from build123d import *

# Parameters (mm, degrees)
F0_R     = 35
F1_DEPTH = 25
F3_DEPTH = 5


with BuildPart() as f1:
    # F0 (on Top) → F1 (new body)
    with BuildSketch(Plane.XY):
        Circle(F0_R)
    extrude(amount=F1_DEPTH)

    # F2 (on face) → F3 (join)
    with BuildSketch(Plane(origin=(0, 0, 0), x_dir=(1, 0, 0), z_dir=(0, 0, -1))):
        with BuildLine():
            Line((-5, 22.5), (-5, 17.811513))
            ThreePointArc((-5, 17.811513), (-18.5, 0), (-5, -17.811513))
            Line((-5, -17.811513), (-5, -22.5))
            Line((-5, -22.5), (5, -22.5))
            Line((5, -22.5), (5, -17.811513))
            ThreePointArc((5, -17.811513), (18.5, 0), (5, 17.811513))
            Line((5, 17.811513), (5, 22.5))
            Line((5, 22.5), (-5, 22.5))
        make_face()
    extrude(amount=F3_DEPTH)


solid = f1.part
Part model, mm, in its own coordinate system. A direction names the side the tool comes from. Round coordinates to 2 decimals unless told otherwise and drop trailing zeros. Order: outer loops, then holes, each group sorted by start corner. A loop starts at its lowest first (then second) coordinate and runs counter-clockwise, first axis right, second up. Notation, with made-up numbers: (-33.5, -26.75) -> (-9.5, -26.75) arc R16 ccw to (-9.5, -20.75) -> close; hole circle Ø1 at (-27, 68). An arc over 180 degrees is marked (long way). Put each result on its own line as item: value.
Q1. Band-saw the part on A-A (x = 0). Give the cut face in (y, z).
From the geometry:
outline: (-35, 0) -> (-22.5, 0) -> (-22.5, -5) -> (22.5, -5) -> (22.5, 0) -> (35, 0) -> (35, 25) -> (-35, 25) -> close
Q2. Tool access for faces 1 (the face through (18.497, 0.336, -2.465)), 2 (the face through (5, -20, -2)), 3 (the face through (-18.497, -0.336, -2.465)), 4 (the face through (-5, 20, -2)), 5 (the face through (-5, -20, -2)): list every direction of +Z, -Z, +X, -X, +Y, -Y with a clear straight run to the whole face (end or side of a thin tool).
From the geometry:
face 1: -Z, +X
face 2: -Z, +X, -Y
face 3: -Z, -X
face 4: -Z, -X, +Y
face 5: -Z, -X, -Y
Q3. Wall check: line 1 (Z direction, x = -9, y = -30); line 2 (Y direction, x = -0.5, z = -2.75); line 3 (Y direction, x = 1, z = 7.25). Give the ranges that are in metal, low to high. Write a range as [from, to].
From the geometry:
line 1: z = [0, 25]
line 2: y = [-22.5, 22.5]
line 3: y = [-34.99, 34.99]
Q4. Band-saw the part on D-D (z = 4). Give the cut face in (x, y).
From the geometry:
outline: circle Ø70 at (0, 0)
Q5. Pin check, flat tips, straight feed: pin 1 Ø10 at (y, z) = (7.5, 0.5) entering from +X; pin 2 Ø5 at (y, z) = (-21, -2) entering from -X; pin 3 Ø8 at (x, z) = (-6.5, 5) entering from -Y. Stop position of each tip, or through.
From the geometry:
pin 1: stops at x = 34.91
pin 2: stops at x = -29.06
pin 3: stops at y = -34.91
Q6. Band-saw the part on B-B (z = -2.25). Give the cut face in (x, y), and give its area (3 significant figures).
From the geometry:
outline: (-5, -22.5) -> (5, -22.5) -> (5, -17.81) arc R18.5 ccw to (5, 17.81) -> (5, 22.5) -> (-5, 22.5) -> (-5, 17.81) arc R18.5 ccw to (-5, -17.81) -> close
area: 1,160 mm2
Q7. Band-saw the part on C-C (y = 27). Give the cut face in (x, z).
From the geometry:
outline: (-22.27, 0) -> (22.27, 0) -> (22.27, 25) -> (-22.27, 25) -> close
